Autodesk Inventor part; units mm, degrees
ref_plane "YZ Plane" through (0, 0, 0) normal (1, 0, 0) x (0, 1, 0)
ref_plane "XZ Plane" through (0, 0, 0) normal (0, 1, 0) x (-1, 0, 0)
ref_plane "XY Plane" through (0, 0, 0) normal (0, 0, 1) x (1, 0, 0)
sketch "Sketch1" plane through (0, 0, 0) normal (0, 1, 0) x (-1, 0, 0)
  line L0 (0, 0) -> (0, -25.4)
  line L1 (0, -25.4) -> (3.175, -25.4)
  line L2 (3.175, -25.4) -> (3.175, -3.175)
  line L3 (3.175, -3.175) -> (25.4, -3.175)
  line L4 (25.4, -3.175) -> (25.4, 0)
  line L5 (25.4, 0) -> (0, 0)
  dimension "d0" = 25.4
  dimension "d1" = 3.175
  dimension "d2" = 22.225
  dimension "d3" = 22.225
extrude "Extrusion1" add sketch "Sketch1" along normal blind 50.8
sketch "Sketch2" plane through (-25.4, 0, 0) normal (0, 0, 1) x (1, 0, 0)
  line L0 (22.225, 0) -> (22.225, 50.8)
  line L1 (22.225, 0) -> (0, 0)
  line L2 (22.225, 50.8) -> (0, 50.8)
  circle A0 centre (14.605, 45.72) radius 1.9304
  circle A1 centre (14.605, 5.08) radius 1.9304
  circle A2 centre (-9.525, 25.4) radius 24.13
  line L3 (25.4, 0) -> (22.225, 0)
  dimension "d9" = 3.8608
  dimension "d10" = 3.8608
extrude "Extrusion2" cut sketch "Sketch2" against normal blind 63.5
sketch "Sketch3" plane through (0, 0, 0) normal (1, 0, 0) x (0, 0, -1)
  line L0 (25.4, 0) -> (25.4, 50.8)
  line L1 (0, 3.2295) -> (0, 47.5705)
  line L2 (0, 50.8) -> (25.4, 50.8)
  line L3 (25.4, 0) -> (3.175, 0)
  circle A0 centre (12.7, 9.525) radius 1.9304
  circle A1 centre (12.7, 41.275) radius 1.9304
  point P0 (0, 0)
  point P1 (12.7, 50.8)
  point P2 (14.2875, 0)
  dimension "d29" = 9.525
  dimension "d30" = 12.7
  dimension "d31" = 9.525
  dimension "d32" = 12.7
  dimension "d33" = 3.8608
  dimension "d34" = 3.8608
extrude "Extrusion3" cut sketch "Sketch3" against normal blind 63.5
properties part number "Frame Bracket"
CAD build for the part. Positions are in the model's coordinates, mm. A direction names the side the tool comes from. Round coordinates to 2 decimals unless told otherwise and drop trailing zeros. Write each loop counter-clockwise with the first axis right and the second up, starting at its lowest first coordinate (ties: lowest second). Pieces come first, ordered by that corner, then holes. Notation, with made-up numbers: (64, 86.5) - (120, 86.5) arc R16 cw to (120, 95.5) - close; hole circle Ø2 at (26.25, -36). An arc over 180 degrees is marked (long way). Write item = value, one per line. Start each with the question number.
Q1. Which spindle directions (+Z, -Z, +X, -X, +Y, -Y) get a long thin tool onto all of the face, cutting with end or side? Do faces 1 (the flat face through (-9, 25, -3.175)), 2 (the cylindrical face through (-1.57, 11.44, -12.45)). Say none if no direction does.
Q2. Band-saw the part on C-C (y = 47). Give the cut face in (x, z) (3 decimals), then the cut area to 3 significant figures.
Q3. Band-saw the part on B-B (z = -12.7). Give the cut face in (x, y) (3 decimals).
Q4. Mould opens along X. For faces 3 (the flat face through (-10, 25, 0)), 4 (the flat face through (-25.4, 49, -2)), 5 (the cylindrical face through (-11.046, 47.634, -1.565)) say: pulls with the +X half, pulls with the -X half, needs draft (parallel to the pull), parting line crosses it, or undercut.
Q5. Band-saw the part on D-D (x = -22.5). Give the cut face in (y, z) (3 decimals).
Q6. Drop flat-ended pins along their axis: pin 1 (4.5 mm diameter, centred on y = 9.525, z = -12.7, fed in from -X) (3 decimals); pin 2 (3.5 mm diameter, centred on y = 41.275, z = -12.7, fed in from -X); pin 3 (2 mm diameter, centred on y = 38.5, z = -4, fed in from -X); pin 4 (11 mm diameter, centred on x = -14, y = 31, fed in from -Z) (3 decimals). Give the stop position or say it passes through.
Q7. Probe L1, parallel to Y at x = -0.85, z = -12.7; L2, parallel to X at y = 12, z = -9.25 (3 decimals). List the from-to ranges inside material, lowest first. Write a range as from..to.
Q8. Band-saw the part on A-A (x = -11.5). Give the cut face in (y, z) (3 decimals), then the cut area to 3 significant figures.
Answers below:
q1.face_1 = -Z, -X, +Y, -Y
q1.face_2 = +X, -X
q2.outline = (-24.169, -3.175) - (-12.24, -3.175) - (-12.24, 0) - (-24.169, 0) - close; (-9.35, -3.175) - (-3.175, -3.175) - (-3.175, -25.4) - (0, -25.4) - (0, 0) - (-9.35, 0) - close
q2.area = 138 mm2
q3.outline = (-3.175, 0) - (0, 0) - (0, 7.595) - (-3.175, 7.595) - close; (-3.175, 11.455) - (0, 11.455) - (0, 39.345) - (-3.175, 39.345) - close; (-3.175, 43.205) - (0, 43.205) - (0, 50.8) - (-3.175, 50.8) - close
q4.face_3 = needs draft
q4.face_4 = pulls with the -X half
q4.face_5 = undercut
q5.outline = (0, -3.175) - (4.715, -3.175) - (4.715, 0) - (0, 0) - close; (46.085, -3.175) - (50.8, -3.175) - (50.8, 0) - (46.085, 0) - close
q6.pin_1 = -3.175
q6.pin_2 = through
q6.pin_3 = -15.04
q6.pin_4 = -3.175
q7.L1 = 0..7.59, 11.46..39.34, 43.21..50.8
q7.L2 = -3.175..0
q8.outline = (0, -3.175) - (3.283, -3.175) - (3.283, 0) - (0, 0) - close; (6.877, -3.175) - (19.61, -3.175) - (19.61, 0) - (6.877, 0) - close; (31.19, -3.175) - (43.923, -3.175) - (43.923, 0) - (31.19, 0) - close; (47.517, -3.175) - (50.8, -3.175) - (50.8, 0) - (47.517, 0) - close
q8.area = 102 mm2
